Geometry: final body of the model. Coordinates: model frame, mm. A direction names the side the tool comes from. Give positions to 0.01 mm unless a question says otherwise; leave off trailing zeros. Write each loop counter-clockwise with the first axis right and the second up, starting at its lowest first coordinate (ties: lowest second). Pieces come first, ordered by that corner, then holes. Notation, with made-up numbers: (87, 47) -> (137, 47) arc R33 cw to (137, 79) -> close; hole circle Ø1 at (-31, -38). An arc over 180 degrees is marked (long way). Answer as a JSON object with one key per item and string values.
Autodesk Inventor part; units mm, degrees
ref_plane "YZ Plane" through (0, 0, 0) normal (1, 0, 0) x (0, 1, 0)
ref_plane "XZ Plane" through (0, 0, 0) normal (0, 1, 0) x (-1, 0, 0)
ref_plane "XY Plane" through (0, 0, 0) normal (0, 0, 1) x (1, 0, 0)
sketch "Sketch1" plane through (0, 0, 0) normal (0, 0, 1) x (1, 0, 0)
  line L0 (787.4, -34.925) -> (547.2722, -34.925) construction
  line L1 (793.75, -30.988) -> (793.75, 781.812) construction
  line L2 (787.4, 785.749) -> (101.6, 785.749) construction
  line L3 (95.25, 781.812) -> (95.25, -30.988) construction
  line L4 (795.3375, -36.5125) -> (93.6625, -36.5125)
  line L5 (93.6625, -36.5125) -> (93.6625, 787.3365)
  line L6 (93.6625, 787.3365) -> (795.3375, 787.3365)
  line L7 (795.3375, 787.3365) -> (795.3375, -36.5125)
  line L8 (877.8875, -119.0625) -> (11.1125, -119.0625)
  line L9 (11.1125, -119.0625) -> (11.1125, 869.8865)
  line L10 (11.1125, 869.8865) -> (877.8875, 869.8865)
  line L11 (877.8875, 869.8865) -> (877.8875, -119.0625)
  point P0 (0, 0)
  dimension "d0" = 1.5875
  dimension "d1" = 1.5875
  dimension "d2" = 1.5875
  dimension "d3" = 1.5875
  dimension "d4" = 82.55
extrude "Extrusion1" add sketch "Sketch1" against normal blind 127
fillet "Fillet1" radius 31.75 8 edges at (444.5, -119.0625, -127) (444.5, -119.0625, 0) (11.1125, 375.412, 0) (11.1125, 375.412, -127) (444.5, 869.8865, -127) (444.5, 869.8865, 0) (877.8875, 375.412, -127) (877.8875, 375.412, 0)
sketch "Sketch2" plane through (0, 0, -127) normal (0, 0, -1) x (-1, 0, 0)
  line L0 (-547.2722, -247.9153) -> (-341.7278, -247.9153)
  line L1 (-341.7278, -247.9153) -> (-341.7278, 127.868)
  line L2 (-341.7278, 127.868) -> (-547.2722, 127.868)
  line L3 (-547.2722, 127.868) -> (-547.2722, -247.9153)
  line L4 (-547.2722, -34.925) -> (-548.4674, -30.988)
  line L5 (-341.7278, -34.925) -> (-340.5326, -30.988)
  point P0 (0, 0)
extrude "Extrusion2" cut sketch "Sketch2" against normal through all
equation "\"d1\" = d0"
equation "\"d2\" = d0"
equation "\"d3\" = d0"
properties part number "BumperSub"
Q1. First-contact query: P1, Ø8, axis at x = 100.5, y = 124, coming from the +Z side; P2, Ø10, axis at x = 107, z = -111.5, coming from the +Y side; P3, Ø5, axis at y = 717, z = -19.5, coming from the +X side. Flat tips, straight axial feed; report the tip coordinate or a pass-through.
Values:
{"P1": "through", "P2": "y = 867.83", "P3": "x = 876.35"}
Q2. Cut plane D-D (x = 482). Return the cut outline in (y, z), and give its area (3 significant figures).
Values:
{"outline": "(787.34, -127) -> (838.14, -127) arc R31.75 ccw to (869.89, -95.25) -> (869.89, -31.75) arc R31.75 ccw to (838.14, 0) -> (787.34, 0) -> close", "area": "10,100 mm²"}
Q3. Material intervals for L1, parallel to X at y = 533, z = -97.5; L2, parallel to X at y = 51, z = -78; L3, parallel to Y at x = 634.5, z = -72, sorted ascending. Write a range as from..to.
Values:
{"L1": "11.19..93.66, 795.34..877.81", "L2": "11.11..93.66, 795.34..877.89", "L3": "-119.06..-36.51, 787.34..869.89"}
Q4. Cut plane A-A (y = 689.5). Return the cut outline in (x, z).
Values:
{"outline": "(11.11, -95.25) arc R31.75 ccw to (42.86, -127) -> (93.66, -127) -> (93.66, 0) -> (42.86, 0) arc R31.75 ccw to (11.11, -31.75) -> close; (795.34, -127) -> (846.14, -127) arc R31.75 ccw to (877.89, -95.25) -> (877.89, -31.75) arc R31.75 ccw to (846.14, 0) -> (795.34, 0) -> close"}
Q5. Cut plane C-C (z = -79). Return the cut outline in (x, y), and give its area (3 significant figures).
Values:
{"outline": "(11.11, -119.06) -> (341.73, -119.06) -> (341.73, -36.51) -> (93.66, -36.51) -> (93.66, 787.34) -> (795.34, 787.34) -> (795.34, -36.51) -> (547.27, -36.51) -> (547.27, -119.06) -> (877.89, -119.06) -> (877.89, 869.89) -> (11.11, 869.89) -> close", "area": "262,000 mm²"}
Q6. Set-up query: faces 4 (the flat face through (673, -36.512, -63)), 5 (the flat face through (179, -119.062, -63)). Return all of +Z, -Z, +X, -X, +Y, -Y with unobstructed straight access to the full face (end or side cutting, diameter ignored); none if empty.
Values:
{"face 4": "+Z, -Z", "face 5": "+Z, -Z, +X, -X, -Y"}
Q7. Cut plane B-B (x = 191). Return the cut outline in (y, z), and give its area (3 significant figures).
Values:
{"outline": "(-119.06, -95.25) arc R31.75 ccw to (-87.31, -127) -> (-36.51, -127) -> (-36.51, 0) -> (-87.31, 0) arc R31.75 ccw to (-119.06, -31.75) -> close; (787.34, -127) -> (838.14, -127) arc R31.75 ccw to (869.89, -95.25) -> (869.89, -31.75) arc R31.75 ccw to (838.14, 0) -> (787.34, 0) -> close", "area": "20,100 mm²"}
Q8. Mould query, pull axis X, two halves, no side actions, for faces 1 (the cylindrical face through (20.66, 382.335, -117.946)), 2 (the flat face through (341.728, -78, -64)), 3 (the flat face through (562, 789, -127)). Classes: pulls with the +X half, pulls with the -X half, needs draft (parallel to the pull), parting line crosses it, or undercut.
Values:
{"face 1": "pulls with the -X half", "face 2": "undercut", "face 3": "needs draft"}
